Read the model definition and answer for the solid it produces. Units are mm, in the model's axes. Coordinates: 2 decimals unless noted, no trailing zeros. Order: outer loops, then holes, each group sorted by start corner. A loop starts at its lowest first (then second) coordinate and runs counter-clockwise, first axis right, second up. Notation, with made-up numbers: M 52.25,55 L 80.25,55 A25 ccw 80.25,93 Z; hole C 26,4.25 d9. An arc over 180 degrees is marked long. Write each question's results on one line, items separated by ' | '.
```python
from build123d import *

# Parameters (mm, degrees)
F0_W     = 260
F0_H     = 940
F1_DEPTH = 5
F2_SIZE  = 9.99999


# Not quite as in the source:
# - a fillet or chamfer is up to 0.001 mm smaller than in the source, because OpenCascade refuses the exact size


with BuildPart() as f1:
    # F0 (on Right) → F1 (new body, symmetric)
    with BuildSketch(Plane.YZ):
        with Locations((130, -470)):
            Rectangle(F0_W, F0_H)
    extrude(amount=F1_DEPTH, both=True)

    # F2 (size 10 in the source; OpenCascade refuses exactly that, so slightly less here)
    f2_edges = [f1.edges().sort_by_distance(p)[0] for p in [
        (5, 0, -470),
        (5, 130, 0),
        (5, 260, -470),
        (5, 130, -940),
    ]]
    chamfer(f2_edges, length=F2_SIZE)


solid = f1.part
```
(1) Given pin 1 (1.5 mm diameter, centred on x = -3, y = 123, fed in from -Z); pin 2 (2 mm diameter, centred on x = -3.5, z = -307, fed in from +Y); pin 3 (1 mm diameter, centred on x = 3, z = -241.5, fed in from +Y), each flat-ended and moving along its own axis, determine where each tip first touches the part or whether it passes through.
Conclusion:
pin 1: z = -938.75 | pin 2: y = 259.5 | pin 3: y = 252.5
(2) The part is cut by section B-B, the plane x = -2. Write down the section's boundary in (y, z).
Conclusion:
outline: M 3,-937 L 257,-937 L 257,-3 L 3,-3 Z
(3) Straight lines are drawn through the part: line 1 (Y direction, x = -0.25, z = -89); line 2 (Z direction, x = 2.5, y = 206); line 3 (Y direction, x = -1.5, z = -631). For each, find the intervals that lie inside material, in ascending order.
Conclusion:
line 1: 4.75 to 255.25 | line 2: -932.5 to -7.5 | line 3: 3.5 to 256.5
